from build123d import *

# Parameters (mm, degrees)
SKETCH1_W           = 300
SKETCH1_H           = 200
BOSS_EXTRUDE1_DEPTH = 5
SKETCH3_W           = 20
SKETCH3_H           = 20
SKETCH3_H_2         = 40
CUT_EXTRUDE1_DEPTH  = 5
CUT_EXTRUDE2_DEPTH  = 10
SKETCH5_W           = 20
SKETCH5_H           = 20
BOSS_EXTRUDE2_DEPTH = 5


with BuildPart() as part:
    # Sketch1 → Boss-Extrude1 (new body)
    with BuildSketch(Plane.XY):
        Rectangle(SKETCH1_W, SKETCH1_H)
    extrude(amount=BOSS_EXTRUDE1_DEPTH)

    # Sketch3 → Cut-Extrude1 (cut)
    with BuildSketch(Plane.XY.offset(5)):
        with Locations((-140, -90)):
            Rectangle(SKETCH3_W, SKETCH3_H)
        with Locations((-140, 80)):
            Rectangle(SKETCH3_W, SKETCH3_H_2)
        with Locations((140, 80)):
            Rectangle(SKETCH3_W, SKETCH3_H_2)
        with Locations((140, -90)):
            Rectangle(SKETCH3_W, SKETCH3_H)
    extrude(amount=-CUT_EXTRUDE1_DEPTH, mode=Mode.SUBTRACT)

    # Sketch4 → Cut-Extrude2 (cut)
    with BuildSketch(Plane.XY.offset(5)):
        with BuildLine():
            Line((-15, -40), (-15, 60))
            Line((-15, 60), (-43.008301528, 100))
            Line((-43.008301528, 100), (43.008301528, 100))
            Line((43.008301528, 100), (15, 60))
            Line((15, 60), (15, -40))
            ThreePointArc((15, -40), (0, -55), (-15, -40))
        make_face()
    extrude(amount=-CUT_EXTRUDE2_DEPTH, mode=Mode.SUBTRACT)

    # Sketch5 → Boss-Extrude2 (add)
    with BuildSketch(Plane.XY.offset(5)):
        with Locations((-140, 70)):
            Rectangle(SKETCH5_W, SKETCH5_H)
    extrude(amount=-BOSS_EXTRUDE2_DEPTH)


solid = part.part
The model under review builds one solid part; all positions refer to its coordinate system, in mm. A direction names the side the tool comes from. Round coordinates to 2 decimals unless told otherwise and drop trailing zeros. Loops run counter-clockwise (first coordinate to the right, second up) from the corner with the lowest first, then second, coordinate; pieces in that order, holes last. Notation, with made-up numbers: M -20,5 L 39,5 A12 cw 39,18 Z; hole C 60,-6 d3. An arc over 180 degrees is marked long. Answer as a JSON object with one key per item and string values.
Item 1: For line 1 along X through (y, z) = (16, 3.9); line 2 along Y through (x, z) = (135, 2.6); line 3 along X through (y, z) = (-88.5, 0.55), list the stretches that pass through material, from the lowest coordinate up.
Check sheet entries:
{"line 1": "-150 to -15, 15 to 150", "line 2": "-80 to 60", "line 3": "-130 to 130"}
Item 2: We need section B-B, the plane z = 2.8. State the section outline as (x, y) points, and give its area (3 significant figures).
Check sheet entries:
{"outline": "M -150,-80 L -130,-80 L -130,-100 L 130,-100 L 130,-80 L 150,-80 L 150,60 L 130,60 L 130,100 L 43.01,100 L 15,60 L 15,-40 A15 cw -15,-40 L -15,60 L -43.01,100 L -130,100 L -130,80 L -150,80 Z", "area": "52,300 mm2"}
Item 3: We need section D-D, the plane y = -50. State the section outline as (x, z) points, and give its area (3 significant figures).
Check sheet entries:
{"outline": "M -150,0 L -11.18,0 L -11.18,5 L -150,5 Z; M 11.18,0 L 150,0 L 150,5 L 11.18,5 Z", "area": "1,390 mm2"}
Item 4: We need section A-A, the plane y = 10. State the section outline as (x, z) points.
Check sheet entries:
{"outline": "M -150,0 L -15,0 L -15,5 L -150,5 Z; M 15,0 L 150,0 L 150,5 L 15,5 Z"}
Item 5: The part is to be moulded in two halves that separate along X. For faces 3 (the face through (-35, 1, 0)), 4 (the face through (-28.81, 79.72, 2.54)), say which applies: +X half, -X half, draft (parallel to the pull), parting line (faces both ways), or undercut.
Check sheet entries:
{"face 3": "draft", "face 4": "undercut"}
Item 6: Tool access review of faces 1 (the face through (29.2, 80.28, 2.54)), 2 (the face through (-35, 1, 5)): name each direction out of +Z, -Z, +X, -X, +Y, -Y from which nothing blocks a thin tool from reaching the whole face with its end or side.
Check sheet entries:
{"face 1": "+Z, -Z, +Y", "face 2": "+Z, +X, -X, +Y, -Y"}
Item 7: Clearance check with flat-ended pins moving along their axes: P1, Ø10, axis at x = -81.5, y = 52.5, coming from the -Z side; P2, Ø1.5, axis at y = 91, z = 2, coming from the -X side; P3, Ø2.5, axis at x = -140.5, z = 3, coming from the -Y side; P4, Ø2.5, axis at y = 74, z = 2.5, coming from the +X side. State where each tip first meets the part, or that it passes through.
Check sheet entries:
{"P1": "z = 0", "P2": "x = -130", "P3": "y = -80", "P4": "x = 130"}
Item 8: We need section C-C, the plane x = 0. State the section outline as (y, z) points.
Check sheet entries:
{"outline": "M -100,0 L -55,0 L -55,5 L -100,5 Z"}
